```python
from build123d import *

# Parameters (mm, degrees)
BOSS_EXTRUDE1_DEPTH = 1.524


with BuildPart() as part:
    # Sketch1 → Boss-Extrude1 (new body)
    with BuildSketch(Plane.XY):
        with BuildLine():
            Line((106.800157748, 0), (106.800157748, -1.524))
            Line((106.800157748, -1.524), (105.60228421, -1.524))
            Line((105.60228421, -1.524), (106.906721504, -4.193201134))
            ThreePointArc((106.906721504, -4.193201134), (104.68375507, -7.107123849), (101.031549593, -6.800659311))
            ThreePointArc((101.031549593, -6.800659311), (97.409591285, -2.343413311), (96.581327911, 3.339860717))
            Line((96.581327911, 3.339860717), (95.016948104, 3.963243569))
            Line((95.016948104, 3.963243569), (95.633020179, 5.509276977))
            Line((95.633020179, 5.509276977), (94.224893193, 6.070395327))
            Line((94.224893193, 6.070395327), (93.642665079, 4.609293369))
            Line((93.642665079, 4.609293369), (92.836519037, 4.930530972))
            ThreePointArc((92.836519037, 4.930530972), (93.215521974, 2.459616544), (93.944606865, 0.068487824))
            Line((93.944606865, 0.068487824), (95.231857751, 0.60397688))
            Line((95.231857751, 0.60397688), (95.633020179, -0.895095706))
            Line((95.633020179, -0.895095706), (94.556110103, -1.331762333))
            ThreePointArc((94.556110103, -1.331762333), (97.492489487, -5.581662211), (101.546965864, -8.782473698))
            Line((101.546965864, -8.782473698), (102.225393513, -7.690984294))
            Line((102.225393513, -7.690984294), (103.519739314, -8.495499643))
            Line((103.519739314, -8.495499643), (102.906411146, -9.482253643))
            ThreePointArc((102.906411146, -9.482253643), (104.901784449, -10.255997053), (106.977037338, -10.77898742))
            ThreePointArc((106.977037338, -10.77898742), (107.562157749, -10.833369035), (108.14727816, -10.77898742))
            ThreePointArc((108.14727816, -10.77898742), (110.222531049, -10.255997053), (112.217904351, -9.482253643))
            Line((112.217904351, -9.482253643), (111.604576184, -8.495499643))
            Line((111.604576184, -8.495499643), (112.898921985, -7.690984294))
            Line((112.898921985, -7.690984294), (113.577349634, -8.782473698))
            ThreePointArc((113.577349634, -8.782473698), (117.631826011, -5.581662211), (120.568205395, -1.331762333))
            Line((120.568205395, -1.331762333), (119.491295318, -0.895095706))
            Line((119.491295318, -0.895095706), (119.892457747, 0.60397688))
            Line((119.892457747, 0.60397688), (121.179708632, 0.068487824))
            ThreePointArc((121.179708632, 0.068487824), (121.908793523, 2.459616544), (122.287796461, 4.930530972))
            Line((122.287796461, 4.930530972), (121.481650419, 4.609293369))
            Line((121.481650419, 4.609293369), (120.899422305, 6.070395327))
            Line((120.899422305, 6.070395327), (119.491295318, 5.509276977))
            Line((119.491295318, 5.509276977), (120.107367394, 3.963243569))
            Line((120.107367394, 3.963243569), (118.542987586, 3.339860717))
            ThreePointArc((118.542987586, 3.339860717), (117.714724213, -2.343413311), (114.092765904, -6.800659311))
            ThreePointArc((114.092765904, -6.800659311), (110.440560427, -7.107123849), (108.217593993, -4.193201134))
            Line((108.217593993, -4.193201134), (109.522031288, -1.524))
            Line((109.522031288, -1.524), (108.32415775, -1.524))
            Line((108.32415775, -1.524), (108.32415775, 0))
            Line((108.32415775, 0), (106.800157748, 0))
        make_face()
    extrude(amount=BOSS_EXTRUDE1_DEPTH)


solid = part.part
```
CAD build for the part. Positions are in the model's coordinates, mm. A direction names the side the tool comes from. Round coordinates to 2 decimals unless told otherwise and drop trailing zeros. Loops run counter-clockwise (first coordinate to the right, second up) from the corner with the lowest first, then second, coordinate; pieces in that order, holes last. Notation, with made-up numbers: (31.25, 24.5) - (82.25, 24.5) arc R13 ccw to (82.25, 49.5) - close; hole circle Ø5 at (49, -13.5). An arc over 180 degrees is marked (long way). Return JSON: item names as keys, results as strings. Group by question number.
Q1. Band-saw the part on D-D on y = -6.5. Give the cut face in (x, z), plus the area to 3 significant figures.
Q2. Band-saw the part on B-B on y = 1.25. Give the cut face in (x, z).
Q3. Band-saw the part on C-C on x = 100.5. Give the cut face in (y, z).
Q4. Band-saw the part on A-A on y = -2. Give the cut face in (x, z), plus the area to 3 significant figures.
Q5. Drill centre lines: line 1 along X through (y, z) = (-7, 1.25); line 2 along X through (y, z) = (0.5, 0.7); line 3 along X through (y, z) = (3, 0.2). Where is each one in solid material? Low to high. Write a range as [from, to].
Q6. Two-plate mould, pull along X, no slides. Class faces 4 (the face through (93.21, 2.49, 0.75)), 5 (the face through (106.245, -2.84, 0.751)), 6 (the face through (121.9, 2.43, 0.75)): +X half, -X half, draft (parallel to the pull), parting line (faces both ways), or undercut.
Q7. Tool access for faces 1 (the face through (95.1, -1.11, 0.75)), 2 (the face through (120.53, 0.34, 0.75)), 3 (the face through (94.9, 5.8, 0.8)): list every direction of +Z, -Z, +X, -X, +Y, -Y with a clear straight run to the whole face (end or side of a thin tool).
Q8. Flat gauge pins, fed straight in: pin 1 Ø0.8 at (y, z) = (-1, 1) entering from +X; pin 2 Ø0.8 at (y, z) = (-1, 1) entering from -X; pin 3 Ø0.8 at (x, z) = (107.5, 1) entering from +Y; pin 4 Ø3 at (x, y) = (101.5, -3.5) entering from +Z. Where does each tip first touch, or does it go through?
Solutions:
{
 "1": {"outline": "(98.42, 0) - (100.63, 0) - (100.63, 1.52) - (98.42, 1.52) - close; (105.64, 0) - (109.49, 0) - (109.49, 1.52) - (105.64, 1.52) - close; (114.49, 0) - (116.7, 0) - (116.7, 1.52) - (114.49, 1.52) - close", "area": "12.6 mm^2"},
 "2": {"outline": "(93.54, 0) - (96.52, 0) - (96.52, 1.52) - (93.54, 1.52) - close; (118.6, 0) - (121.59, 0) - (121.59, 1.52) - (118.6, 1.52) - close"},
 "3": {"outline": "(-8.13, 0) - (-6.4, 0) - (-6.4, 1.52) - (-8.13, 1.52) - close"},
 "4": {"outline": "(94.9, 0) - (97.27, 0) - (97.27, 1.52) - (94.9, 1.52) - close; (105.83, 0) - (109.29, 0) - (109.29, 1.52) - (105.83, 1.52) - close; (117.86, 0) - (120.22, 0) - (120.22, 1.52) - (117.86, 1.52) - close", "area": "12.5 mm^2"},
 "5": {"line 1": "x = [98.99, 101.37], [104.91, 110.22], [113.76, 116.13]", "line 2": "x = [93.78, 94.98], [95.26, 96.6], [118.52, 119.86], [120.14, 121.34]", "line 3": "x = [93.1, 96.54], [118.58, 122.02]"},
 "6": {"face 4": "-X half", "face 5": "undercut", "face 6": "+X half"},
 "7": {"face 1": "+Z, -Z, -X", "face 2": "+Z, -Z", "face 3": "+Z, -Z, +Y"},
 "8": {"pin 1": "stops at x = 120.57", "pin 2": "stops at x = 94.56", "pin 3": "stops at y = 0", "pin 4": "passes through"}
}
